from build123d import *

# Parameters (mm, degrees)
SKETCH_R       = 14.25
PAD_DEPTH      = 29
SKETCH001_R    = 2.1
HOLE_DEPTH     = 12
HOLE_TIPS_R    = 2.1
SKETCH002_R    = 2.1
HOLE001_DEPTH  = 12
HOLE001_TIPS_R = 2.1
CHAMFER_SIZE   = 0.5


with BuildPart() as part:
    # Sketch → Pad (new body)
    with BuildSketch(Plane.XY):
        with BuildLine():
            Line((-29, 23.5), (29, 23.5))
            ThreePointArc((30, 22.5), (29.707107, 23.207107), (29, 23.5))
            Line((30, 22.5), (30, 0))
            ThreePointArc((29.330127, -2.5), (29.829629, -1.294095), (30, 0))
            Line((20.092523, -18.5), (29.330127, -2.5))
            ThreePointArc((15.762396, -21), (18.262396, -20.330127), (20.092523, -18.5))
            Line((-15.762396, -21), (15.762396, -21))
            ThreePointArc((-20.092523, -18.5), (-18.262396, -20.330127), (-15.762396, -21))
            Line((-29.330127, -2.5), (-20.092523, -18.5))
            ThreePointArc((-30, 0), (-29.829629, -1.294095), (-29.330127, -2.5))
            Line((-30, 22.5), (-30, 0))
            ThreePointArc((-29, 23.5), (-29.707107, 23.207107), (-30, 22.5))
        make_face()
        Circle(SKETCH_R, mode=Mode.SUBTRACT)
    extrude(amount=PAD_DEPTH)

    # Sketch001 (on Face14 of Pad) → Hole (cut)
    with BuildSketch(Plane(origin=(0, 0, 0), x_dir=(1, 0, 0), z_dir=(0, 0, -1))):
        with Locations((-19, 0)):
            Circle(SKETCH001_R)
        with Locations((-13.435029, 13.435029)):
            Circle(SKETCH001_R)
        with Locations((13.435029, 13.435029)):
            Circle(SKETCH001_R)
        with Locations((19, 0)):
            Circle(SKETCH001_R)
        with Locations((13.435029, -13.435029)):
            Circle(SKETCH001_R)
        with Locations((-13.435029, -13.435029)):
            Circle(SKETCH001_R)
    extrude(amount=-HOLE_DEPTH, mode=Mode.SUBTRACT)

    # Hole tips → Hole tip 1 section 0
    with BuildSketch(Plane(origin=(0, 0, 12), x_dir=(1, 0, 0), z_dir=(0, 0, -1)), mode=Mode.PRIVATE) as hole_tip_1_s0:
        with Locations((-19, 0)):
            Circle(HOLE_TIPS_R)
    loft([hole_tip_1_s0.sketch, Vertex(-19, 0, 13.261807)], mode=Mode.SUBTRACT)

    # Hole tips → Hole tip 2 section 0
    with BuildSketch(Plane(origin=(0, 0, 12), x_dir=(1, 0, 0), z_dir=(0, 0, -1)), mode=Mode.PRIVATE) as hole_tip_2_s0:
        with Locations((-13.435029, 13.435029)):
            Circle(HOLE_TIPS_R)
    loft([hole_tip_2_s0.sketch, Vertex(-13.435029, -13.435029, 13.261807)], mode=Mode.SUBTRACT)

    # Hole tips → Hole tip 3 section 0
    with BuildSketch(Plane(origin=(0, 0, 12), x_dir=(1, 0, 0), z_dir=(0, 0, -1)), mode=Mode.PRIVATE) as hole_tip_3_s0:
        with Locations((13.435029, 13.435029)):
            Circle(HOLE_TIPS_R)
    loft([hole_tip_3_s0.sketch, Vertex(13.435029, -13.435029, 13.261807)], mode=Mode.SUBTRACT)

    # Hole tips → Hole tip 4 section 0
    with BuildSketch(Plane(origin=(0, 0, 12), x_dir=(1, 0, 0), z_dir=(0, 0, -1)), mode=Mode.PRIVATE) as hole_tip_4_s0:
        with Locations((19, 0)):
            Circle(HOLE_TIPS_R)
    loft([hole_tip_4_s0.sketch, Vertex(19, 0, 13.261807)], mode=Mode.SUBTRACT)

    # Hole tips → Hole tip 5 section 0
    with BuildSketch(Plane(origin=(0, 0, 12), x_dir=(1, 0, 0), z_dir=(0, 0, -1)), mode=Mode.PRIVATE) as hole_tip_5_s0:
        with Locations((13.435029, -13.435029)):
            Circle(HOLE_TIPS_R)
    loft([hole_tip_5_s0.sketch, Vertex(13.435029, 13.435029, 13.261807)], mode=Mode.SUBTRACT)

    # Hole tips → Hole tip 6 section 0
    with BuildSketch(Plane(origin=(0, 0, 12), x_dir=(1, 0, 0), z_dir=(0, 0, -1)), mode=Mode.PRIVATE) as hole_tip_6_s0:
        with Locations((-13.435029, -13.435029)):
            Circle(HOLE_TIPS_R)
    loft([hole_tip_6_s0.sketch, Vertex(-13.435029, 13.435029, 13.261807)], mode=Mode.SUBTRACT)

    # Sketch002 (on Face2 of Hole) → Hole001 (cut)
    with BuildSketch(Plane(origin=(0, 23.5, 0), x_dir=(-1, 0, 0), z_dir=(0, 1, 0))):
        with Locations((-25, 5)):
            Circle(SKETCH002_R)
        with Locations((25, 5)):
            Circle(SKETCH002_R)
        with Locations((-25, 24)):
            Circle(SKETCH002_R)
        with Locations((25, 24)):
            Circle(SKETCH002_R)
    extrude(amount=-HOLE001_DEPTH, mode=Mode.SUBTRACT)

    # Hole001 tips → Hole001 tip 1 section 0
    with BuildSketch(Plane(origin=(0, 11.5, 0), x_dir=(-1, 0, 0), z_dir=(0, 1, 0)), mode=Mode.PRIVATE) as hole001_tip_1_s0:
        with Locations((-25, 5)):
            Circle(HOLE001_TIPS_R)
    loft([hole001_tip_1_s0.sketch, Vertex(25, 10.238193, 5)], mode=Mode.SUBTRACT)

    # Hole001 tips → Hole001 tip 2 section 0
    with BuildSketch(Plane(origin=(0, 11.5, 0), x_dir=(-1, 0, 0), z_dir=(0, 1, 0)), mode=Mode.PRIVATE) as hole001_tip_2_s0:
        with Locations((25, 5)):
            Circle(HOLE001_TIPS_R)
    loft([hole001_tip_2_s0.sketch, Vertex(-25, 10.238193, 5)], mode=Mode.SUBTRACT)

    # Hole001 tips → Hole001 tip 3 section 0
    with BuildSketch(Plane(origin=(0, 11.5, 0), x_dir=(-1, 0, 0), z_dir=(0, 1, 0)), mode=Mode.PRIVATE) as hole001_tip_3_s0:
        with Locations((-25, 24)):
            Circle(HOLE001_TIPS_R)
    loft([hole001_tip_3_s0.sketch, Vertex(25, 10.238193, 24)], mode=Mode.SUBTRACT)

    # Hole001 tips → Hole001 tip 4 section 0
    with BuildSketch(Plane(origin=(0, 11.5, 0), x_dir=(-1, 0, 0), z_dir=(0, 1, 0)), mode=Mode.PRIVATE) as hole001_tip_4_s0:
        with Locations((25, 24)):
            Circle(HOLE001_TIPS_R)
    loft([hole001_tip_4_s0.sketch, Vertex(-25, 10.238193, 24)], mode=Mode.SUBTRACT)

    # Chamfer
    chamfer_edges = [part.edges().sort_by_distance(p)[0] for p in [
        (-14.25, 0, 0),
        (-16.9, 0, 0),
        (-11.335029, -13.435029, 0),
        (-11.335029, 13.435029, 0),
        (15.535029, -13.435029, 0),
        (21.1, 0, 0),
        (15.535029, 13.435029, 0),
        (0, 23.5, 0),
        (0, 23.5, 29),
        (-27.1, 23.5, 24),
        (22.9, 23.5, 24),
        (22.9, 23.5, 5),
        (-27.1, 23.5, 5),
        (-14.25, 0, 29),
    ]]
    chamfer(chamfer_edges, length=CHAMFER_SIZE)


solid = part.part
Build history of the part. All positions in model axes, mm. A direction names the side the tool comes from. Coordinates: 2 decimals unless noted, no trailing zeros. Order: outer loops, then holes, each group sorted by start corner. A loop starts at its lowest first (then second) coordinate and runs counter-clockwise, first axis right, second up. Notation, with made-up numbers: (-19.75, -30.75) - (5.25, -30.75) arc R25 ccw to (5.25, -13.75) - close; hole circle Ø3 at (61, 43). An arc over 180 degrees is marked (long way). Write item = value, one per line. Start each with the question number.
1) Saw through at B-B on x = 0. Write the cut outline in (y, z).
2) Saw through at A-A on y = 20.5. Write the cut outline in (x, z), then the cut area to 3 significant figures.
3) Flat gauge pins, fed straight in: pin 1 Ø12 at (x, z) = (16.5, 16.5) entering from -Y; pin 2 Ø5 at (x, z) = (25, 24) entering from -Y; pin 3 Ø5 at (x, z) = (-25, 5) entering from +Y; pin 4 Ø5 at (x, y) = (19, 0) entering from -Z. Where does each tip first touch, or does it go through?
4) Two-plate mould, pull along Y, no slides. Class faces 3 (the face through (23.87, 17.33, 25.77)), 4 (the face through (-13.12, 13.33, 13.06)), 5 (the face through (24.56, -10.26, 28.75)): pulls with the +Y half, pulls with the -Y half, needs draft (parallel to the pull), parting line crosses it, or undercut.
5) Wall check: line 1 along X through (y, z) = (20.5, 5.25); line 2 along X through (y, z) = (-0.5, 3.75); line 3 along X through (y, z) = (3.5, 12.75). Give the ranges that are in metal, low to high. Write a range as from..to.
6) Saw through at C-C on z = 20. Write the cut outline in (x, y), then the cut area to 3 significant figures.
7) 3-axis set-ups, long thin cutter, end or side, ignore diameter. For faces 1 (the face through (29.825, -1.312, 14.304)), 2 (the face through (21.003, -0.631, 6.17)): which of +Z, -Z, +X, -X, +Y, -Y reach the whole face in a straight line?
8) Saw through at D-D on z = 9.25. Write the cut outline in (x, y), then the cut area to 3 significant figures.
From the geometry:
q1.outline = (-21, 0.5) - (-20.5, 0) - (-14.75, 0) - (-14.25, 0.5) - (-14.25, 28.5) - (-14.75, 29) - (-20.5, 29) - (-21, 28.5) - close; (14.25, 0.5) - (14.75, 0) - (23, 0) - (23.5, 0.5) - (23.5, 28.5) - (23, 29) - (14.75, 29) - (14.25, 28.5) - close
q2.outline = (-30, 0.5) - (-29.5, 0) - (29.5, 0) - (30, 0.5) - (30, 28.5) - (29.5, 29) - (-29.5, 29) - (-30, 28.5) - close; hole circle Ø4.2 at (-25, 5); hole circle Ø4.2 at (-25, 24); hole circle Ø4.2 at (25, 5); hole circle Ø4.2 at (25, 24)
q2.area = 1,680 mm^2
q3.pin_1 = -21
q3.pin_2 = -14.33
q3.pin_3 = 23.4
q3.pin_4 = 0.1
q4.face_3 = needs draft
q4.face_4 = undercut
q4.face_5 = pulls with the -Y half
q5.line_1 = -30..-27.09, -22.91..22.91, 27.09..30
q5.line_2 = -29.97..-21.04, -16.96..-14.24, 14.24..16.96, 21.04..29.97
q5.line_3 = -30..-13.81, 13.81..30
q6.outline = (-30, 0) arc R5 ccw to (-29.33, -2.5) - (-20.09, -18.5) arc R5 ccw to (-15.76, -21) - (15.76, -21) arc R5 ccw to (20.09, -18.5) - (29.33, -2.5) arc R5 ccw to (30, 0) - (30, 22.5) arc R1 ccw to (29, 23.5) - (-29, 23.5) arc R1 ccw to (-30, 22.5) - close; hole circle Ø28.5 at (0, 0)
q6.area = 1,810 mm^2
q7.face_1 = +Z, -Z, +X, -Y
q7.face_2 = -Z
q8.outline = (-30, 0) arc R5 ccw to (-29.33, -2.5) - (-20.09, -18.5) arc R5 ccw to (-15.76, -21) - (15.76, -21) arc R5 ccw to (20.09, -18.5) - (29.33, -2.5) arc R5 ccw to (30, 0) - (30, 22.5) arc R1 ccw to (29, 23.5) - (-29, 23.5) arc R1 ccw to (-30, 22.5) - close; hole circle Ø4.2 at (-19, 0); hole circle Ø4.2 at (-13.44, -13.44); hole circle Ø4.2 at (-13.44, 13.44); hole circle Ø28.5 at (0, 0); hole circle Ø4.2 at (13.44, -13.44); hole circle Ø4.2 at (13.44, 13.44); hole circle Ø4.2 at (19, 0)
q8.area = 1,720 mm^2
